```python
from build123d import *

# Parameters (mm, degrees)
F3_R            = 225
F4_DEPTH        = 160
F5_R            = 140
F6_DEPTH        = 25
F7_R            = 25
F8_DEPTH        = 7
F8_COPIES_COUNT = 5
F9_R            = 10
F10_DEPTH       = 10


# Not quite as in the source:
# - a pattern or mirror of a feature is missing from the dataset's text; its kind, count and spacing are read off the source's solid


with BuildPart() as f4:
    # F3 (on Right) → F4 (new body)
    with BuildSketch(Plane.YZ):
        Circle(F3_R)
    extrude(amount=F4_DEPTH)

    # F5 (on face) → F6 (cut)
    with BuildSketch(Plane.YZ.offset(160)):
        Circle(F5_R)
    extrude(amount=-F6_DEPTH, mode=Mode.SUBTRACT)

    # F7 (on face) → F8 (cut)
    with BuildSketch(Plane.YZ.offset(135)):
        with Locations((85, 0)):
            Circle(F7_R)
    f8 = extrude(amount=-F8_DEPTH, mode=Mode.SUBTRACT)

    # F8_copies: F8 ×5 about axis
    f8_copies_axis = Axis((0, 0, 0), (1, 0, 0))
    for i in range(1, F8_COPIES_COUNT):
        add(f8.rotate(f8_copies_axis, i * 360 / F8_COPIES_COUNT), mode=Mode.SUBTRACT)

    # F9 (on face) → F10 (join)
    with BuildSketch(Plane.YZ.offset(135)):
        Circle(F9_R)
    extrude(amount=F10_DEPTH)


solid = f4.part
```
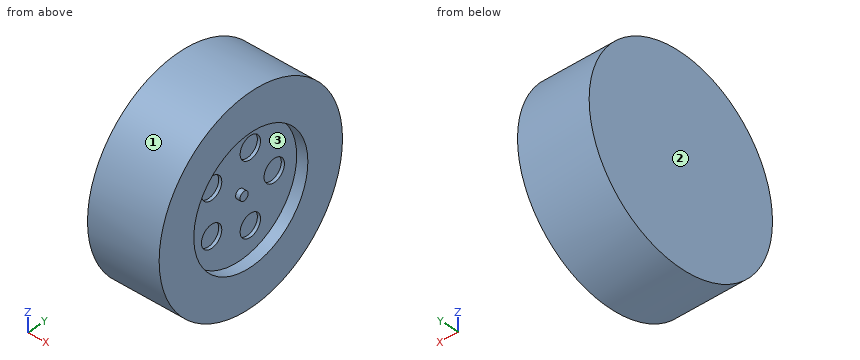
Check sheet for the modelled part. Datum: model origin and axes. Units: mm. Face numbers are marked on the shaded views. Give positions to 0.01 mm unless a question says otherwise; leave off trailing zeros. Write each loop counter-clockwise with the first axis right and the second up, starting at its lowest first coordinate (ties: lowest second). Pieces come first, ordered by that corner, then holes.
Item 1: Scan lines: L1, parallel to Z at x = 153, y = 0; L2, parallel to X at y = -31.5, z = 84; L3, parallel to Z at x = 146, y = -101.5. Record each from-to range of solid material in increasing order.
Item 2: Gauge pin test, flat ends, axial feed: pin 1 (6 mm diameter, centred on x = 121.5, z = 23, fed in from +Y); pin 2 (2 mm diameter, centred on x = 101.5, y = -29, fed in from +Z); pin 3 (3 mm diameter, centred on x = 87.5, z = -144.5, fed in from +Y); pin 4 (6 mm diameter, centred on y = -29, z = -95.5, fed in from -X). Record the tip position at first contact, or that the pin passes through.
Item 3: Cross-section at D-D (z = -180). Enter the section's corners in (x, y).
Item 4: Cross-section at C-C (x = 83.5). Enter the section's corners in (y, z).
Item 5: Cross-section at A-A (z = 0). Enter the section's corners in (x, y).
Item 6: Cross-section at B-B (y = 92). Enter the section's corners in (x, z).
Item 7: Draft check along Z on the marked faces 1, 2 and 3. Enter one of: released by +Z, released by -Z, zero draft, split by the parting line, or undercut.
Report:
1. L1: z = -225 to -140, 140 to 225
1. L2: x = 0 to 135
1. L3: z = -200.81 to -96.42, 96.42 to 200.81
2. pin 1: stops at y = 224.11
2. pin 2: stops at z = 223.25
2. pin 3: stops at y = 173.71
2. pin 4: stops at x = 0
3. outline: (0, -135) - (160, -135) - (160, 135) - (0, 135) - close
4. outline: circle Ø450 at (0, 0)
5. outline: (0, -225) - (160, -225) - (160, -140) - (135, -140) - (135, -10) - (145, -10) - (145, 10) - (135, 10) - (135, 60) - (128, 60) - (128, 110) - (135, 110) - (135, 140) - (160, 140) - (160, 225) - (0, 225) - close
6. outline: (0, -205.33) - (160, -205.33) - (160, -105.53) - (135, -105.53) - (135, -24) - (128, -24) - (128, 24) - (135, 24) - (135, 105.53) - (160, 105.53) - (160, 205.33) - (0, 205.33) - close
7. face 1: split by the parting line
7. face 2: zero draft
7. face 3: undercut
